CAD build for the part. Positions are in the model's coordinates, mm. Face numbers are marked on the shaded views. A direction names the side the tool comes from. Give positions to 0.01 mm unless a question says otherwise; leave off trailing zeros. Write each loop counter-clockwise with the first axis right and the second up, starting at its lowest first coordinate (ties: lowest second). Pieces come first, ordered by that corner, then holes. Notation, with made-up numbers: (-20.75, 51.5) - (13.25, 51.5) arc R12 cw to (13.25, 61.5) - close; hole circle Ø11 at (27, 84). An arc over 180 degrees is marked (long way). Put each result on its own line as item: value. Start each with the question number.
1. Drop flat-ended pins along their axis: pin 1 (8.5 mm diameter, centred on x = 14.29, z = 11.52, fed in from +Y); pin 2 (1.6 mm diameter, centred on y = -1.5, z = 25, fed in from +X); pin 3 (3 mm diameter, centred on x = 35, z = 33.5, fed in from +Y). Give the stop position or say it passes through.
2. Cut at A-A on z = 35. List the corners of the cut face in (x, y).
3. Cut at B-B on y = -1.5. List the corners of the cut face in (x, z).
4. Tool access for the marked faces 1 and 2: list every direction of +Z, -Z, +X, -X, +Y, -Y with a clear straight run to the whole face (end or side of a thin tool).
5. Mould opens along X. For the marked faces 3 and 4 say: +X half, -X half, draft (parallel to the pull), parting line (faces both ways), or undercut.
6. Wall check: line 1 (Z direction, x = 17, y = -5); line 2 (Z direction, x = 17, y = -5.5); line 3 (X direction, y = -2, z = 7). Give the ranges that are in metal, low to high.
7. Cut at C-C on x = 16. Give the number of separate pieces and of enclosed holes in the cut face, and give its area (3 significant figures).
8. Cut at D-D on x = 32.5. List the corners of the cut face in (y, z), and give its area (3 significant figures).
from build123d import *

# Parameters (mm, degrees)
BOSS_EXTRU_1_DEPTH                             = 60
CONG_1_R                                       = 1
FRAISAGE_POUR_VIS_T_TE_FRAIS_E_M62_D           = 6.6
FRAISAGE_POUR_VIS_T_TE_FRAIS_E_M62_DEPTH       = 8
FRAISAGE_POUR_VIS_T_TE_FRAIS_E_M62_CSINK_D     = 12.6
FRAISAGE_POUR_VIS_T_TE_FRAIS_E_M62_CSINK_ANGLE = 90
FRAISAGE_POUR_VIS_T_TE_FRAIS_E_M62_TIP         = 1.982840043


with BuildPart() as part:
    # Esquisse1 → Boss.-Extru.1 (new body)
    with BuildSketch(Plane.XY):
        Polygon((0, 0), (28, 0), (28, -3.1), (53, -3.1), (53, -6.2), (0, -6.2), align=None)
    extrude(amount=BOSS_EXTRU_1_DEPTH)

    # Congé1
    cong_1_edges = [part.edges().sort_by_distance(p)[0] for p in [
        (53, -3.1, 30),
        (53, -6.2, 30),
    ]]
    fillet(cong_1_edges, radius=CONG_1_R)

    # Fraisage pour vis à tête fraisée M62
    with Locations(Plane(origin=(0, -6.2, 0), x_dir=(-1, 0, 0), z_dir=(0, -1, 0))):
        with Locations((-14.293755616, -11.515144287), (-14.293755616, -47.158937793)):
            CounterSinkHole(FRAISAGE_POUR_VIS_T_TE_FRAIS_E_M62_D / 2, FRAISAGE_POUR_VIS_T_TE_FRAIS_E_M62_CSINK_D / 2, depth=FRAISAGE_POUR_VIS_T_TE_FRAIS_E_M62_DEPTH, counter_sink_angle=FRAISAGE_POUR_VIS_T_TE_FRAIS_E_M62_CSINK_ANGLE)
            with Locations((0, 0, -(FRAISAGE_POUR_VIS_T_TE_FRAIS_E_M62_DEPTH + FRAISAGE_POUR_VIS_T_TE_FRAIS_E_M62_TIP / 2))):  # 118° drill point
                Cone(0, FRAISAGE_POUR_VIS_T_TE_FRAIS_E_M62_D / 2, FRAISAGE_POUR_VIS_T_TE_FRAIS_E_M62_TIP, mode=Mode.SUBTRACT)


solid = part.part
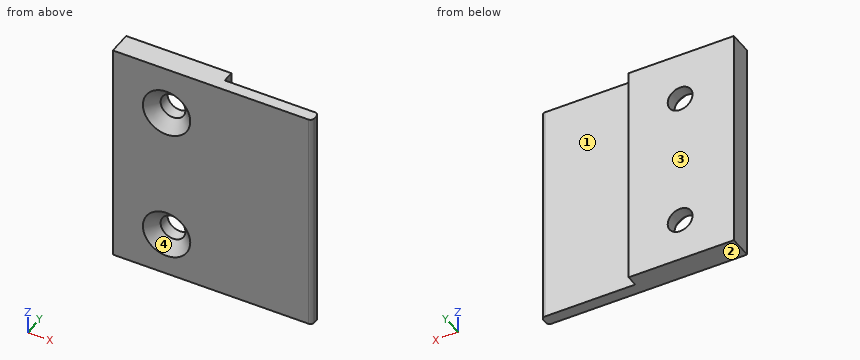
Report:
1. pin 1: stops at y = 0
1. pin 2: stops at x = 28
1. pin 3: stops at y = -3.1
2. outline: (0, -6.2) - (52, -6.2) arc R1 ccw to (53, -5.2) - (53, -4.1) arc R1 ccw to (52, -3.1) - (28, -3.1) - (28, 0) - (0, 0) - close
3. outline: (0, 0) - (28, 0) - (28, 60) - (0, 60) - close; hole circle Ø6.6 at (14.29, 11.52); hole circle Ø6.6 at (14.29, 47.16)
4. face 1: +Z, -Z, +X, +Y
4. face 2: -Z, +X, -X, +Y, -Y
5. face 3: draft
5. face 4: undercut
6. line 1: z = 0 to 7.19, 15.84 to 42.84, 51.48 to 60
6. line 2: z = 0 to 6.61, 16.42 to 42.26, 52.06 to 60
6. line 3: x = 0 to 28
7. separate pieces: 3
7. enclosed holes: 0
7. area: 282 mm²
8. outline: (-6.2, 0) - (-3.1, 0) - (-3.1, 60) - (-6.2, 60) - close
8. area: 186 mm²
